Could you check a few things on this model? Use its own coordinates, in mm. A direction names the side the tool comes from. Coordinates: 2 decimals unless noted, no trailing zeros. Write each loop counter-clockwise with the first axis right and the second up, starting at its lowest first coordinate (ties: lowest second). Pieces come first, ordered by that corner, then holes.
```python
from build123d import *
from build123d.topology import SkipClean

# Parameters (mm, degrees)
SKETCH_1_W               = 12
SKETCH_1_H               = 15
SKETCH_1_R               = 0.8
SKETCH_1_R_2             = 3
EXTRUDE_1_DEPTH          = 2
EXTRUDE_3_DEPTH          = 12
CUT_EXTRUDE_1_REACH      = 17.37
SKETCH_2_3_R             = 1.5
CUT_EXTRUDE_2_DEPTH      = 3
CUT_EXTRUDE_2_DEPTH_BACK = 3
FILLET_1_R               = 2


with BuildPart() as part:
    # 草图1 → 凸台-拉伸1 (new body)
    with BuildSketch(Plane(origin=(0, 0, 0), x_dir=(1, 0, 0), z_dir=(0, 1, 0))):
        Rectangle(SKETCH_1_W, SKETCH_1_H)
        with Locations(Location((-4.5, 2.5, 0), (0, 0, 270))):
            Circle(SKETCH_1_R, mode=Mode.SUBTRACT)
        with Locations(Location((4.5, 2.5, 0), (0, 0, 270))):
            Circle(SKETCH_1_R, mode=Mode.SUBTRACT)
        with Locations(Location((0, 2.5, 0), (0, 0, 270))):
            Circle(SKETCH_1_R_2, mode=Mode.SUBTRACT)
    extrude(amount=EXTRUDE_1_DEPTH)

    # 草图2 → 凸台-拉伸3 (add)
    with BuildSketch(Plane.ZY.offset(6)):
        with BuildLine():
            ThreePointArc((7.5, 3), (4.5, 6), (1.5, 3))
            Line((1.5, 3), (1.5, 2))
            Line((1.5, 2), (3.381966011, 2))
            ThreePointArc((3.381966011, 2), (3.964766865, 4.401258538), (6, 3))
            ThreePointArc((6, 3), (5.901258538, 2.464766865), (5.618033989, 2))
            Line((5.618033989, 2), (7.5, 2))
            Line((7.5, 2), (7.5, 3))
        make_face()
    extrude(amount=-EXTRUDE_3_DEPTH)

    # 草图2<3> → 切除-拉伸1 (cut, up to next)
    with BuildSketch(Plane.ZY.offset(6), mode=Mode.PRIVATE) as cut_extrude_1_sk1:
        with Locations((4.5, 3)):
            Circle(SKETCH_2_3_R)
    cut_extrude_1_tool1 = extrude(cut_extrude_1_sk1.sketch, amount=-CUT_EXTRUDE_1_REACH, mode=Mode.PRIVATE) & part.part
    add(cut_extrude_1_tool1.solids().sort_by_distance((-6, 3, 4.5))[0], mode=Mode.SUBTRACT)

    # 草图5 → 切除-拉伸2 (cut, two sides: drawn at the far end of the back side and taken through both)
    with SkipClean():  # the faces are left unmerged after this step: merging them gives an invalid solid
        with BuildSketch(Plane.ZY.offset(-CUT_EXTRUDE_2_DEPTH_BACK)):
            with BuildLine():
                Line((1.5, 2), (1.5, 0))
                Line((1.5, 0), (7.5, 0))
                Line((7.5, 0), (7.5, 3))
                ThreePointArc((7.5, 3), (4.5, 6), (1.5, 3))
                Line((1.5, 3), (1.5, 2))
            make_face()
        extrude(amount=CUT_EXTRUDE_2_DEPTH + CUT_EXTRUDE_2_DEPTH_BACK, mode=Mode.SUBTRACT)

    # 圆角1
    fillet_1_edges = [part.edges().sort_by_distance(p)[0] for p in [
        (-4.5, 0, 7.5),
        (4.5, 0, 7.5),
    ]]
    fillet(fillet_1_edges, radius=FILLET_1_R)


solid = part.part
```
1. I want a section at A-A on z = -2.5. Please give me the cut outline in (x, y), plus the area to 3 significant figures.
Verdict:
outline: (-6, 0) - (-5.3, 0) - (-5.3, 2) - (-6, 2) - close; (-3.7, 0) - (-3, 0) - (-3, 2) - (-3.7, 2) - close; (3, 0) - (3.7, 0) - (3.7, 2) - (3, 2) - close; (5.3, 0) - (6, 0) - (6, 2) - (5.3, 2) - close
area: 5.60 mm2
2. I want a section at C-C on y = 2.2. Please give me the cut outline in (x, z), plus the area to 3 significant figures.
Verdict:
outline: (-6, 1.5) - (-3, 1.5) - (-3, 3.23) - (-6, 3.23) - close; (-6, 5.77) - (-3, 5.77) - (-3, 7.5) - (-6, 7.5) - close; (3, 1.5) - (6, 1.5) - (6, 3.23) - (3, 3.23) - close; (3, 5.77) - (6, 5.77) - (6, 7.5) - (3, 7.5) - close
area: 20.8 mm2
3. If we mould it in two halves opening along X, with no side actions, what happens to faces 1 (the face through (-5.28, 0.99, -2.67)), 2 (the face through (-6, 2, 2)), 3 (the face through (-1.4, 0, 0.4))? For each: pulls with the +X half, pulls with the -X half, needs draft (parallel to the pull), parting line crosses it, or undercut.
Verdict:
face 1: undercut
face 2: pulls with the -X half
face 3: needs draft
4. On a 3-axis mill with a long thin cutter (end or side, diameter ignored), from which of +Z, -Z, +X, -X, +Y, -Y can I reach the whole of each face in a straight line? I mean faces 4 (the face through (-3, 2, 3)), 5 (the face through (4.5, 2.5, 1.5)), 6 (the face through (-4.48, 0.6, 6.93)). Say none if no direction works.
Verdict:
face 4: +Z, +Y, -Y
face 5: -Z, +X, -X, +Y
face 6: +Z, +X, -X, -Y
5. Please list where these lines run through material, in increasing order: line 1 along X through (y, z) = (1.25, -2.5); line 2 along Y through (x, z) = (-3.65, 4.5); line 3 along X through (y, z) = (1.8, 3.5).
Verdict:
line 1: x = -6 to -5.3, -3.7 to -3, 3 to 3.7, 5.3 to 6
line 2: y = 0 to 1.5, 4.5 to 6
line 3: x = -6 to -3, 3 to 6
6. I want a section at B-B on x = 4.5. Please give me the cut outline in (y, z), plus the area to 3 significant figures.
Verdict:
outline: (0, -7.5) - (2, -7.5) - (2, -3.3) - (0, -3.3) - close; (0, -1.7) - (2, -1.7) - (2, 1.5) - (3, 1.5) arc R3 ccw to (3, 7.5) - (2, 7.5) arc R2 ccw to (0, 5.5) - close; hole circle Ø3 at (3, 4.5)
area: 39.0 mm2
7. I want a section at D-D on x = -1.75. Please give me the cut outline in (y, z).
Verdict:
outline: (0, -7.5) - (2, -7.5) - (2, -4.94) - (0, -4.94) - close; (0, -0.06) - (2, -0.06) - (2, 1.5) - (0, 1.5) - close
8. For pin 1 (1.4 mm diameter, centred on x = 4.5, z = -2.5, fed in from -Y); pin 2 (0.5 mm diameter, centred on x = 5, y = 2.5, fed in from -Z); pin 3 (1.6 mm diameter, centred on x = 0, y = 0.5, fed in from +Z), each with a flat end and sliding along its axis, tell me the tip position at first contact or that it passes through.
Verdict:
pin 1: passes through
pin 2: stops at z = 1.5
pin 3: stops at z = 1.5
